Could you check a few things on this drawing? It's one solid part, dimensions in mm from its lowest x, y, z. A direction names the side the tool comes from. Give positions to 0.01 mm unless a question says otherwise; leave off trailing zeros. Loops run counter-clockwise (first coordinate to the right, second up) from the corner with the lowest first, then second, coordinate; pieces in that order, holes last. Notation, with made-up numbers: M 11,68.5 L 61,68.5 A20 cw 61,97.5 Z; hole C -26,42.5 d6. An arc over 180 degrees is marked long. Return JSON: item names as keys, results as strings. Group by question number.
1. If we section it at B-B (y = 9.2): Write out the boundary of the cut face in (x, z).
2. Please list where these lines run through material, in increasing order: line 1 (X direction, y = 1.3, z = 20); line 2 (X direction, y = 11.75, z = 21.5); line 3 (Y direction, x = 20.25, z = 5).
3. If we section it at A-A (x = 9): Write out the boundary of the cut face in (y, z).
4. If we section it at C-C (z = 20): Write out the boundary of the cut face in (x, y), plus the area to 3 significant figures.
5. For the marked faces 1, 2 and 3, which set-ups out of +Z, -Z, +X, -X, +Y, -Y let a thin tool reach every point of the face, with its end or its side?
6. If we mould it in two halves opening along Z, with no side actions, what happens to the marked faces 4, 5 and 6? For each: +Z half, -Z half, draft (parallel to the pull), parting line (faces both ways), or undercut.
7. For pin 1 (9 mm diameter, centred on x = 10, z = 15, fed in from +Y); pin 2 (2.5 mm diameter, centred on x = 33, y = 2, fed in from +Z); pin 3 (4 mm diameter, centred on x = 35.5, y = 1.5, fed in from -Z); pin 4 (3 mm diameter, centred on x = 6, z = 20.5, fed in from -Y), each with a flat end and sliding along its axis, tell me the tip position at first contact or that it passes through.
8. If we section it at D-D (z = 35): Write out the boundary of the cut face in (x, y).
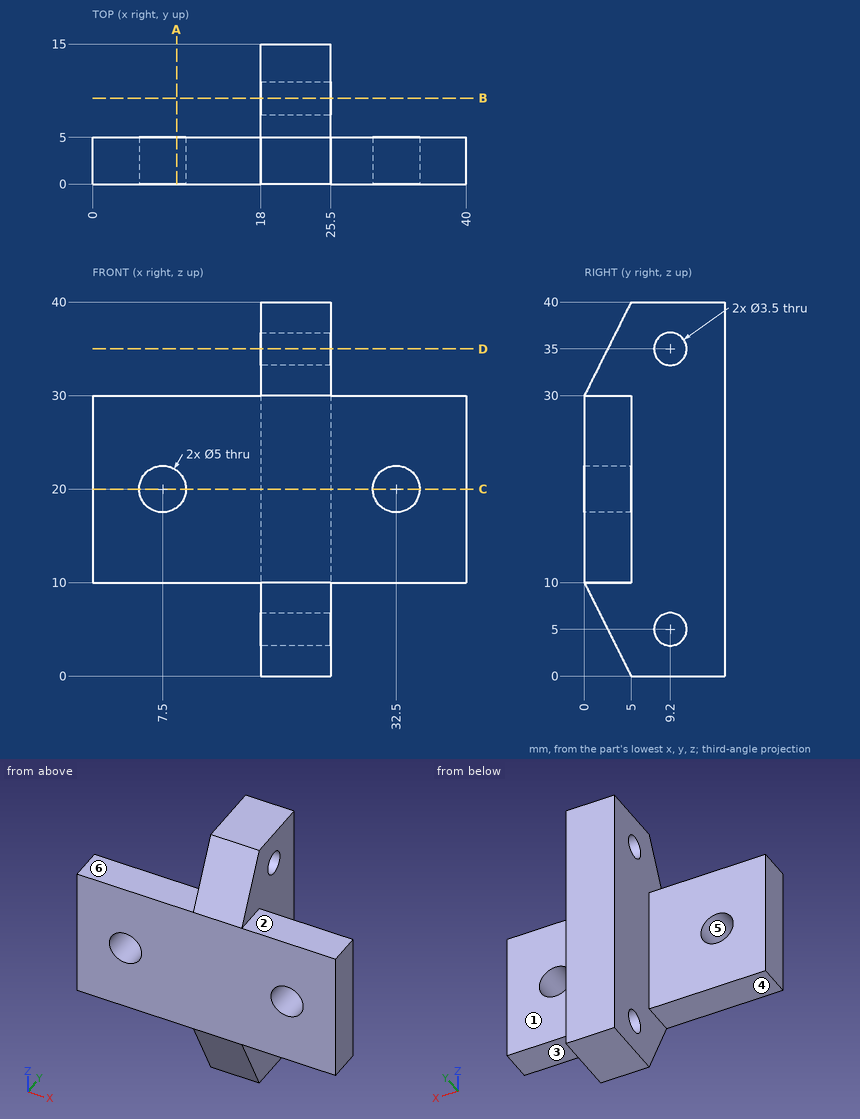
Answer:
{
 "1": {"outline": "M 18,0 L 25.5,0 L 25.5,3.25 L 18,3.25 Z; M 18,6.75 L 25.5,6.75 L 25.5,33.25 L 18,33.25 Z; M 18,36.75 L 25.5,36.75 L 25.5,40 L 18,40 Z"},
 "2": {"line 1": "x = 0 to 5, 10 to 30, 35 to 40", "line 2": "x = 18 to 25.5", "line 3": "y = 2.5 to 7.45, 10.95 to 15"},
 "3": {"outline": "M 0,10 L 5,10 L 5,18 L 0,18 Z; M 0,22 L 5,22 L 5,30 L 0,30 Z"},
 "4": {"outline": "M 0,0 L 5,0 L 5,5 L 0,5 Z; M 10,0 L 30,0 L 30,5 L 25.5,5 L 25.5,15 L 18,15 L 18,5 L 10,5 Z; M 35,0 L 40,0 L 40,5 L 35,5 Z", "area": "225 mm²"},
 "5": {"face 1": "+Z, -Z, +X, +Y", "face 2": "+Z, +X, +Y, -Y", "face 3": "-Z, +X, +Y, -Y"},
 "6": {"face 4": "-Z half", "face 5": "undercut", "face 6": "+Z half"},
 "7": {"pin 1": "stops at y = 5", "pin 2": "stops at z = 30", "pin 3": "stops at z = 10", "pin 4": "stops at y = 0"},
 "8": {"outline": "M 18,2.5 L 25.5,2.5 L 25.5,7.45 L 18,7.45 Z; M 18,10.95 L 25.5,10.95 L 25.5,15 L 18,15 Z"}
}
